Could you check a few things on this drawing? It's one solid part, dimensions in mm from its lowest x, y, z. A direction names the side the tool comes from. Coordinates: 2 decimals unless noted, no trailing zeros. Order: outer loops, then holes, each group sorted by start corner. A loop starts at its lowest first (then second) coordinate and runs counter-clockwise, first axis right, second up. Notation, with made-up numbers: (3, 80.5) - (55, 80.5) arc R5 cw to (55, 87.5) - close; hole circle Ø1 at (59, 86). An arc over 180 degrees is marked (long way). Return JSON: item names as keys, results as strings. Group by question number.
1) Which directions (+Z, -Z, +X, -X, +Y, -Y) give clear straight access to the entire face, cutting with the end or side of a thin tool? Please do the marked faces 1 and 2.
2) For pin 1 Ø1 at (x, z) = (456, 29.5) entering from +Y; pin 2 Ø1 at (x, z) = (410.5, 211.5) entering from -Y, each with a flat end and sliding along its axis, tell me the tip position at first contact or that it passes through.
3) If I drill on line 1 along Z through (x, y) = (248.5, 11); line 2 along X through (y, z) = (11.5, 197); line 3 along Y through (x, z) = (439.5, 46), over which ranges is the centre line in solid material (lowest first)?
4) Imagine slicing it at A-A (x = 241.5). Write out the boundary of the cut face in (y, z).
5) Imagine slicing it at B-B (z = 77.5). Write out the boundary of the cut face in (x, y).
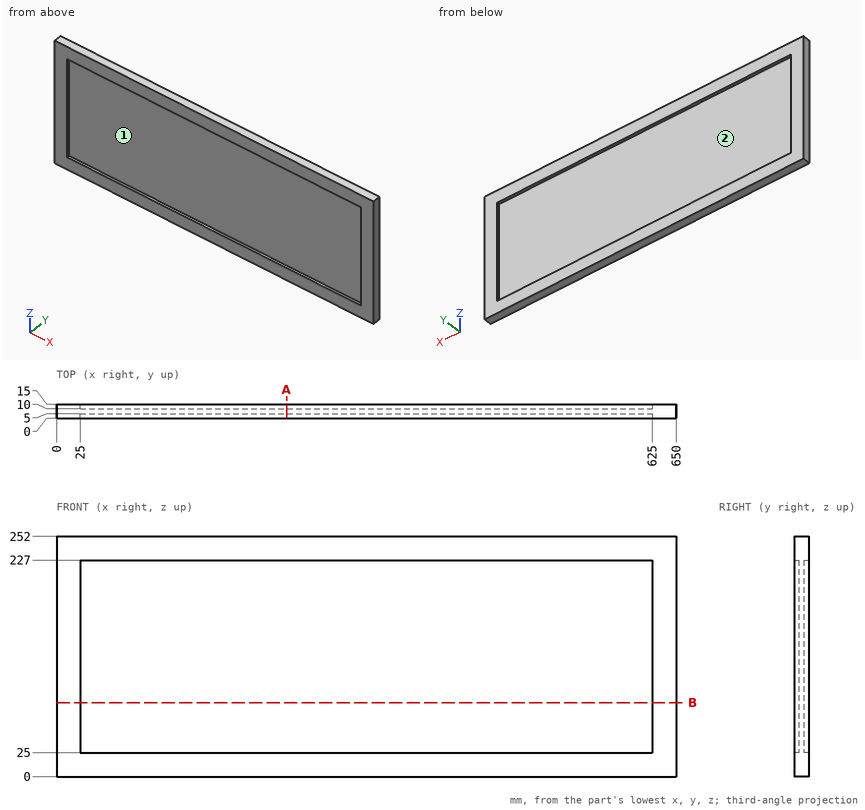
Calculated:
{
 "1": {"face 1": "-Y", "face 2": "+Y"},
 "2": {"pin 1": "y = 10", "pin 2": "y = 5"},
 "3": {"line 1": "0 to 25, 227 to 252", "line 2": "0 to 25, 625 to 650", "line 3": "5 to 10"},
 "4": {"outline": "(0, 0) - (15, 0) - (15, 25) - (10, 25) - (10, 227) - (15, 227) - (15, 252) - (0, 252) - (0, 227) - (5, 227) - (5, 25) - (0, 25) - close"},
 "5": {"outline": "(0, 0) - (25, 0) - (25, 5) - (625, 5) - (625, 0) - (650, 0) - (650, 15) - (625, 15) - (625, 10) - (25, 10) - (25, 15) - (0, 15) - close"}
}
